For this review, take the finished solid that the model builds, in its own axes (mm). A direction names the side the tool comes from. Give positions to 0.01 mm unless a question says otherwise; leave off trailing zeros. Loops run counter-clockwise (first coordinate to the right, second up) from the corner with the lowest first, then second, coordinate; pieces in that order, holes last. Notation, with made-up numbers: (36, -39.75) -> (60, -39.75) arc R14 ccw to (60, -31.75) -> close; hole circle Ø7 at (39.25, 20.25). An arc over 180 degrees is marked (long way). Answer as CSV lines item,"result". Start each with the question number.
Item 1: Clearance check with flat-ended pins moving along their axes: P1, Ø12, axis at x = 64.5, y = -8, coming from the +Z side; P2, Ø3, axis at y = 19, z = 45, coming from the -X side. State where each tip first meets the part, or that it passes through.
Item 2: The part is to be moulded in two halves that separate along X. For faces 1 (the face through (0, 1, 50)), 2 (the face through (20, -1, 45)), 3 (the face through (68.482, 35.067, 10.656)), say which applies: +X half, -X half, draft (parallel to the pull), parting line (faces both ways), or undercut.
Item 3: Add section A-A on z = 20. State the section outline as (x, y) points, plus the area to 3 significant figures.
Item 4: Add section D-D on y = 47. State the section outline as (x, z) points.
Item 5: Machinability: for faces 4 (the face through (-20, -1, 45)), 5 (the face through (-74.04, -42.76, 27.33)), 6 (the face through (-87.871, -52.482, 19.72)), 7 (the face through (57, 1, 40)), which of the approach directions +Z, -Z, +X, -X, +Y, -Y give a long, thin tool a straight path to every point of the face, cutting with its end or side? Answer none if there is none.
Item 6: For L1, parallel to X at y = 35, z = 31.25; L2, parallel to Y at x = 70, z = 20; L3, parallel to X at y = -33, z = 12, list the stretches that pass through material, from the lowest coordinate up. Write a range as from..to.
Item 7: Add section C-C on x = 32.5. State the section outline as (y, z) points, plus the area to 3 significant figures.
Item 8: Add section B-B on y = 18.5. State the section outline as (x, z) points.
```python
from build123d import *

# Parameters (mm, degrees)
BOSS_EXTRUDE3_DEPTH    = 40
M20_TAPPED_HOLE1_D     = 17.5
M20_TAPPED_HOLE1_DEPTH = 25
M20_TAPPED_HOLE1_TIP   = 5.257530416
SKETCH6_W              = 40
SKETCH6_H              = 120
BOSS_EXTRUDE4_DEPTH    = 10


with BuildPart() as part:
    # Sketch1 → Boss-Extrude3 (new body)
    with BuildSketch(Plane.XY):
        with BuildLine():
            Line((70, 60), (-70, 60))
            ThreePointArc((-70, 60), (-87.67766953, 52.67766953), (-95, 35))
            Line((-95, 35), (-95, -35))
            ThreePointArc((-95, -35), (-87.67766953, -52.67766953), (-70, -60))
            Line((-70, -60), (70, -60))
            ThreePointArc((70, -60), (87.67766953, -52.67766953), (95, -35))
            Line((95, -35), (95, 35))
            ThreePointArc((95, 35), (87.67766953, 52.67766953), (70, 60))
        make_face()
    extrude(amount=BOSS_EXTRUDE3_DEPTH)

    # M20 Tapped Hole1
    with Locations(Plane(origin=(-70, 35, 40), x_dir=(1, 0, 0), z_dir=(0, 0, 1))):
        with Locations((0, 0), (0, -70), (140, -70), (140, 0)):
            Hole(M20_TAPPED_HOLE1_D / 2, depth=M20_TAPPED_HOLE1_DEPTH)
            with Locations((0, 0, -(M20_TAPPED_HOLE1_DEPTH + M20_TAPPED_HOLE1_TIP / 2))):  # 118° drill point
                Cone(0, M20_TAPPED_HOLE1_D / 2, M20_TAPPED_HOLE1_TIP, mode=Mode.SUBTRACT)

    # Sketch6 → Boss-Extrude4 (add)
    with BuildSketch(Plane.XY.offset(40)):
        Rectangle(SKETCH6_W, SKETCH6_H)
    extrude(amount=BOSS_EXTRUDE4_DEPTH)


solid = part.part
```
Computed values:
1,P1,"z = 40"
1,P2,"x = -20"
2,face 1,"draft"
2,face 2,"+X half"
2,face 3,"undercut"
3,outline,"(-95, -35) arc R25 ccw to (-70, -60) -> (70, -60) arc R25 ccw to (95, -35) -> (95, 35) arc R25 ccw to (70, 60) -> (-70, 60) arc R25 ccw to (-95, 35) -> close; hole circle Ø17.5 at (-70, -35); hole circle Ø17.5 at (-70, 35); hole circle Ø17.5 at (70, -35); hole circle Ø17.5 at (70, 35)"
3,area,"21,300 mm²"
4,outline,"(-91.93, 0) -> (91.93, 0) -> (91.93, 40) -> (20, 40) -> (20, 50) -> (-20, 50) -> (-20, 40) -> (-91.93, 40) -> close"
5,face 4,"+Z, -X, +Y, -Y"
5,face 5,"+Z"
5,face 6,"+Z, -Z, -X, -Y"
5,face 7,"+Z, +X, +Y, -Y"
6,L1,"-95..-78.75, -61.25..61.25, 78.75..95"
6,L2,"-60..-43.75, -26.25..26.25, 43.75..60"
6,L3,"-95..-73.18, -66.82..66.82, 73.18..95"
7,outline,"(-60, 0) -> (60, 0) -> (60, 40) -> (-60, 40) -> close"
7,area,"4,800 mm²"
8,outline,"(-95, 0) -> (95, 0) -> (95, 40) -> (20, 40) -> (20, 50) -> (-20, 50) -> (-20, 40) -> (-95, 40) -> close"
